Geometry: final body of the model. Coordinates: model frame, mm. Give positions to 0.01 mm unless a question says otherwise; leave off trailing zeros. Order: outer loops, then holes, each group sorted by start corner. A loop starts at its lowest first (then second) coordinate and runs counter-clockwise, first axis right, second up. Notation, with made-up numbers: (25, -19.75) -> (80, -19.75) arc R21 ccw to (80, 4.25) -> close; hole circle Ø7 at (-32.75, -4.75). An arc over 180 degrees is marked (long way). Answer in a Markdown table with one row per item. Add a question column.
Q1. Cut plane C-C on z = 164. Return the cut outline in (x, y), and give its area (3 significant figures).
Q2. Pull-direction query (X, two-part tool) for faces 1 (the face through (122.79, 2.54, -131.48)), 2 (the face through (60.075, 2.465, 190.764)), 3 (the face through (3, 5, -3)), 4 (the face through (124.97, 2.54, -133.82)); classes: +X half, -X half, draft (parallel to the pull), parting line (faces both ways), or undercut.
Q3. Cut plane A-A on y = 2.6. Count the separate pieces of the cut face and the enclosed holes in it, and give its area (3 significant figures).
Q4. Cut plane B-B on x = -99. Return the cut outline in (y, z).
Q5. Contact query for flat-ended pins moving along their axis: P1, Ø7, axis at x = 175, z = 0, coming from the -Y side; P2, Ø3, axis at x = 41, y = 1, coming from the -Z side; P3, Ø4, axis at x = 0, z = 187, coming from the -Y side; P4, Ø3, axis at x = -59, y = 4, coming from the +Z side. Output: stop coordinate, or through.
Q6. Line query: line 1 along X through (y, z) = (3.4, -125); line 2 along X through (y, z) = (0.95, 77.5); line 3 along X through (y, z) = (3.3, -175). Output: solid intervals per line, ascending. Write a range as from..to.
from build123d import *

# Parameters (mm, degrees)
SKETCH_1_R               = 200
EXTRUDE_257_DEPTH        = 5
CUT_EXTRUDE_3_REACH      = 284.887
SKETCH_2_R               = 2.6
PATTERN_CIRCULAR_1_COUNT = 4
SKETCH_4_W               = 3.2
SKETCH_4_H               = 12.2
CUT_REVOLVE_3_ANGLE      = 8.5
FILLET_2_R               = 1.5
CUT_EXTRUDE_1561_REACH   = 284.887
FILLET_1_R               = 1.5


with BuildPart() as part:
    # Sketch 1 → Extrude 257 (new body)
    with BuildSketch(Plane(origin=(0, 0, 0), x_dir=(1, 0, 0), z_dir=(0, 1, 0))):
        with Locations(Location((0, 0, 0), (0, 0, 270))):
            Circle(SKETCH_1_R)
    extrude(amount=EXTRUDE_257_DEPTH)

    # Sketch 2 → Cut-Extrude 3 (cut, up to next)
    with BuildSketch(Plane(origin=(0, 5, 0), x_dir=(1, 0, 0), z_dir=(0, 1, 0)), mode=Mode.PRIVATE) as cut_extrude_3_sk1:
        with Locations(Location((0, -175, 0), (0, 0, 270))):
            Circle(SKETCH_2_R)
    cut_extrude_3_tool1 = extrude(cut_extrude_3_sk1.sketch, amount=-CUT_EXTRUDE_3_REACH, mode=Mode.PRIVATE) & part.part
    # Sketch 2 → Cut-Extrude 3 (cut, up to next)
    with BuildSketch(Plane(origin=(0, 5, 0), x_dir=(1, 0, 0), z_dir=(0, 1, 0)), mode=Mode.PRIVATE) as cut_extrude_3_sk2:
        with Locations(Location((0, -187, 0), (0, 0, 270))):
            Circle(SKETCH_2_R)
    cut_extrude_3_tool2 = extrude(cut_extrude_3_sk2.sketch, amount=-CUT_EXTRUDE_3_REACH, mode=Mode.PRIVATE) & part.part
    cut_extrude_3_1 = cut_extrude_3_tool1.solids().sort_by_distance((0, 5, 175))[0]
    add(cut_extrude_3_1, mode=Mode.SUBTRACT)
    cut_extrude_3_2 = cut_extrude_3_tool2.solids().sort_by_distance((0, 5, 187))[0]
    add(cut_extrude_3_2, mode=Mode.SUBTRACT)
    cut_extrude_3 = cut_extrude_3_1 + cut_extrude_3_2  # Cut-Extrude 3 as one shape, for the pattern or mirror that repeats it

    # Pattern Circular 1: Cut-Extrude 3 ×4 about axis
    pattern_circular_1_axis = Axis((0, 0, 0), (0, 1, 0))
    for i in range(1, PATTERN_CIRCULAR_1_COUNT):
        add(cut_extrude_3.rotate(pattern_circular_1_axis, i * 360 / PATTERN_CIRCULAR_1_COUNT), mode=Mode.SUBTRACT)

    # Sketch 4 → Cut-Revolve 3 (revolve, cut)
    with BuildSketch(Plane(origin=(0, 0, 0), x_dir=(0.73135370161917, 0, -0.6819983600624991), z_dir=(0.6819983600624991, 0, 0.73135370161917))):
        with Locations((181.5, 3)):
            Rectangle(SKETCH_4_W, SKETCH_4_H)
    revolve(axis=Axis((0, -55, 0), (0, 1, 0)), revolution_arc=CUT_REVOLVE_3_ANGLE, mode=Mode.SUBTRACT)

    # Fillet 2
    fillet_2_edges = [part.edges().sort_by_distance(p)[0] for p in [
        (113.982429968, 2.5, -143.29555352),
        (111.990383131, 2.5, -140.791207418),
    ]]
    fillet(fillet_2_edges, radius=FILLET_2_R)

    # Sketch 6 → Cut-Extrude 1561 (cut, up to next)
    with BuildSketch(Plane(origin=(0, 5, 0), x_dir=(1, 0, 0), z_dir=(0, 1, 0)), mode=Mode.PRIVATE) as cut_extrude_1561_sk1:
        with BuildLine():
            Line((127.646791587, 118.032637546), (138.809893683, 128.343047734))
            ThreePointArc((138.809893683, 128.343047734), (139.99182369, 127.052799206), (141.161761211, 125.751666622))
            Line((141.161761211, 125.751666622), (129.820417839, 115.637649754))
            ThreePointArc((129.820417839, 115.637649754), (128.739174201, 116.840198367), (127.646791587, 118.032637546))
        make_face()
    cut_extrude_1561_tool1 = extrude(cut_extrude_1561_sk1.sketch, amount=-CUT_EXTRUDE_1561_REACH, mode=Mode.PRIVATE) & part.part
    add(cut_extrude_1561_tool1.solids().sort_by_distance((134.437436, 5, -122.011787))[0], mode=Mode.SUBTRACT)

    # Fillet 1
    fillet_1_edges = [part.edges().sort_by_distance(p)[0] for p in [
        (129.820417839, 2.5, -115.637649754),
        (127.646791587, 2.5, -118.032637546),
        (138.809893683, 2.5, -128.343047734),
        (141.161761211, 2.5, -125.751666622),
    ]]
    fillet(fillet_1_edges, radius=FILLET_1_R)


solid = part.part
Completed:
| question | item | result |
|---|---|---|
| 1 | outline | (-114.47, 0) -> (114.47, 0) -> (114.47, 5) -> (-114.47, 5) -> close |
| 1 | area | 1,140 mm² |
| 2 | face 1 | undercut |
| 2 | face 2 | parting line |
| 2 | face 3 | draft |
| 2 | face 4 | undercut |
| 3 | separate pieces | 1 |
| 3 | enclosed holes | 10 |
| 3 | area | 125,000 mm² |
| 4 | outline | (0, -173.78) -> (5, -173.78) -> (5, 173.78) -> (0, 173.78) -> close |
| 5 | P1 | stops at y = 0 |
| 5 | P2 | stops at z = -196.06 |
| 5 | P3 | passes through |
| 5 | P4 | stops at z = 191.56 |
| 6 | line 1 | x = -156.12..129.38, 133.79..135.19, 140.26..156.12 |
| 6 | line 2 | x = -184.37..184.37 |
| 6 | line 3 | x = -96.82..-2.6, 2.6..96.82 |
